Autodesk Inventor part; units mm, degrees
ref_plane "YZ Plane" through (0, 0, 0) normal (1, 0, 0) x (0, 1, 0)
ref_plane "XZ Plane" through (0, 0, 0) normal (0, 1, 0) x (-1, 0, 0)
ref_plane "XY Plane" through (0, 0, 0) normal (0, 0, 1) x (1, 0, 0)
sketch "Sketch1" plane through (0, 0, 0) normal (0, 1, 0) x (-1, 0, 0)
  line L0 (-78.994, -44.958) -> (78.994, -44.958)
  line L1 (78.994, -44.958) -> (78.994, 44.958)
  line L2 (78.994, 44.958) -> (-78.994, 44.958)
  line L3 (-78.994, 44.958) -> (-78.994, -44.958)
  line L4 (-78.994, -44.958) -> (78.994, 44.958) construction
  line L5 (78.994, -44.958) -> (-78.994, 44.958) construction
  point P0 (0, 0)
  dimension "d0" = 89.916
  dimension "d1" = 157.988
extrude "Extrusion1" add sketch "Sketch1" along normal blind 55.118
fillet "Fillet1" radius 7.62 4 edges at (78.994, 27.559, 44.958) (78.994, 27.559, -44.958) (-78.994, 27.559, 44.958) (-78.994, 27.559, -44.958)
shell "Shell1" thickness 3.556 removed faces 1 at (23.7913, 55.118, -14.986)
sketch "Sketch2" plane through (-71.374, 3.556, 41.402) normal (0, 1, 0) x (1, 0, 0)
  line L0 (0, 0) -> (142.748, 0)
  line L1 (137.922, 0) -> (137.922, 82.804)
  line L2 (0, 82.804) -> (142.748, 82.804)
  line L3 (4.826, 82.804) -> (4.826, 0)
  line L4 (142.748, 0) -> (0, 0)
  line L5 (-4.064, 4.064) -> (-4.064, 78.74)
  line L6 (146.812, 78.74) -> (146.812, 4.064)
  arc A0 (0, 82.804) -> (-4.064, 78.74) centre (0, 78.74) ccw
  line L7 (-4.064, 78.74) -> (-4.064, 4.064)
  arc A1 (-4.064, 4.064) -> (0, 0) centre (0, 4.064) ccw
  line L8 (0, 0) -> (142.748, 0)
  arc A2 (142.748, 0) -> (146.812, 4.064) centre (142.748, 4.064) ccw
  line L9 (146.812, 4.064) -> (146.812, 78.74)
  arc A3 (146.812, 78.74) -> (142.748, 82.804) centre (142.748, 78.74) ccw
  line L10 (142.748, 82.804) -> (0, 82.804)
  point P0 (71.374, 41.402)
  point P1 (4.826, 0)
  point P2 (0, 82.804)
  point P3 (-4.064, 78.74)
  dimension "d6" = 133.096
  dimension "d7" = 8.89
  dimension "d8" = 8.89
extrude "Extrusion2" add sketch "Sketch2" along normal up to surface (51.562 mm away) contours A1 L5 A0 L2 L3 L0 | L1 L2 A3 L6 A2 L0
equation "\"d7\" = d8"
properties part number "project_box"
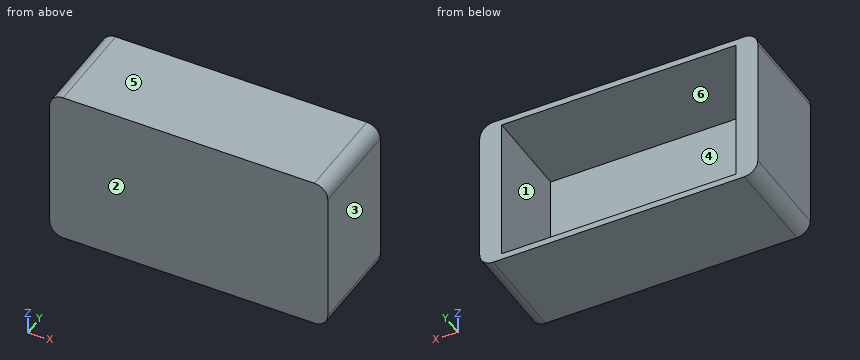
Source: CAD feature listing. Evaluate the final solid. Frame: model axes, mm. Face numbers are marked on the shaded views. A direction names the side the tool comes from. Round coordinates to 2 decimals unless told otherwise and drop trailing zeros. Order: outer loops, then holes, each group sorted by start corner. A loop starts at its lowest first (then second) coordinate and runs counter-clockwise, first axis right, second up. Notation, with made-up numbers: (71, 10.25) -> (79, 10.25) arc R29 cw to (79, 30.25) -> close; hole circle Ø4 at (27.25, 53). An arc over 180 degrees is marked (long way). Answer as CSV lines item,"result".
Item 1: Section A-A, the plane y = 27. Return loops of the section in (x, z), plus the area to 3 significant figures.
A:
outline,"(-78.99, -37.34) arc R7.62 ccw to (-71.37, -44.96) -> (71.37, -44.96) arc R7.62 ccw to (78.99, -37.34) -> (78.99, 37.34) arc R7.62 ccw to (71.37, 44.96) -> (-71.37, 44.96) arc R7.62 ccw to (-78.99, 37.34) -> close; hole (-66.55, -41.4) -> (66.55, -41.4) -> (66.55, 41.4) -> (-66.55, 41.4) -> close"
area,"3,130 mm²"
Item 2: Reachability of the marked faces 5 and 6 from +Z, -Z, +X, -X, +Y, -Y: full face, straight path, thin tool, end or side. Return the list, or none.
A:
face 5,"+Z, +X, -X, +Y, -Y"
face 6,"+Y"
Item 3: Line query: L1, parallel to X at y = 38, z = 22.5; L2, parallel to Z at x = -30, y = 19.5; L3, parallel to Y at x = -52, z = 9. Output: solid intervals per line, ascending.
A:
L1,"-78.99 to -66.55, 66.55 to 78.99"
L2,"-44.96 to -41.4, 41.4 to 44.96"
L3,"0 to 3.56"
Item 4: Pull-direction query (X, two-part tool) for the marked faces 1, 2, 3 and 4; classes: pulls with the +X half, pulls with the -X half, needs draft (parallel to the pull), parting line crosses it, or undercut.
A:
face 1,"undercut"
face 2,"needs draft"
face 3,"pulls with the +X half"
face 4,"undercut"
Item 5: Section C-C, the plane z = 21. Return loops of the section in (x, y), plus the area to 3 significant figures.
A:
outline,"(-78.99, 0) -> (78.99, 0) -> (78.99, 55.12) -> (66.55, 55.12) -> (66.55, 3.56) -> (-66.55, 3.56) -> (-66.55, 55.12) -> (-78.99, 55.12) -> close"
area,"1,850 mm²"
Item 6: Section B-B, the plane x = -34.5. Return loops of the section in (y, z), plus the area to 3 significant figures.
A:
outline,"(0, -44.96) -> (55.12, -44.96) -> (55.12, -41.4) -> (3.56, -41.4) -> (3.56, 41.4) -> (55.12, 41.4) -> (55.12, 44.96) -> (0, 44.96) -> close"
area,"686 mm²"
Item 7: Pin query (flat end, axial travel): pin 1 Ø8 at (x, z) = (-59, 0) entering from -Y. Return the tip coordinate at first contact, or that it passes through.
A:
pin 1,"y = 0"
